from build123d import *

# Parameters (mm, degrees)
SKETCH042_R       = 4
PAD018_DEPTH      = 18.8
SKETCH045_R       = 3.3
PAD019_DEPTH      = 8
SKETCH050_R       = 4
PAD021_DEPTH      = 33.8
CYLINDER003_R     = 3.3
CYLINDER003_DEPTH = 8


with BuildPart() as part:
    # Sketch042 (on DatumPlane) → Pad018 (new body)
    with BuildSketch(Plane(origin=(0, 0, 18.8), x_dir=(0, 1, 0), z_dir=(0, 0, 1))):
        Circle(SKETCH042_R)
    extrude(amount=-PAD018_DEPTH)

    # Sketch045 (on Face2 of Pad018) → Pad019 (join)
    with BuildSketch(Plane(origin=(0, 0, 18.8), x_dir=(0, 1, 0), z_dir=(0, 0, 1))):
        Circle(SKETCH045_R)
    extrude(amount=PAD019_DEPTH)

    # Sketch050 (on Face3 of Pad019) → Pad021 (join)
    with BuildSketch(Plane.YX):
        Circle(SKETCH050_R)
    extrude(amount=PAD021_DEPTH)

    # Cylinder003 → Cylinder003 (join)
    with BuildSketch(Plane.YX.offset(33.8)):
        Circle(CYLINDER003_R)
    extrude(amount=CYLINDER003_DEPTH)


solid = part.part
Can you work these out from the model? Positions are in its coordinate system, mm. A direction names the side the tool comes from. Give positions to 0.01 mm unless a question says otherwise; leave off trailing zeros. Loops run counter-clockwise (first coordinate to the right, second up) from the corner with the lowest first, then second, coordinate; pieces in that order, holes last. Notation, with made-up numbers: (10, 0.25) - (29, 0.25) arc R27 ccw to (29, 31.25) - close; hole circle Ø11 at (7, -34). An arc over 180 degrees is marked (long way). Return JSON: item names as keys, results as strings.
1. I want a section at A-A on x = 0. Please give me the cut outline in (y, z), and give its area (3 significant figures).
Output values:
{"outline": "(-4, -33.8) - (-3.3, -33.8) - (-3.3, -41.8) - (3.3, -41.8) - (3.3, -33.8) - (4, -33.8) - (4, 18.8) - (3.3, 18.8) - (3.3, 26.8) - (-3.3, 26.8) - (-3.3, 18.8) - (-4, 18.8) - close", "area": "526 mm²"}
2. I'm going to push flat-ended pins straight in: pin 1 Ø3 at (y, z) = (-2.5, 4.5) entering from -X; pin 2 Ø3 at (x, z) = (-2, -25) entering from -Y. Where does each tip first touch, or does it pass through?
Output values:
{"pin 1": "stops at x = -3.87", "pin 2": "stops at y = -3.97"}
3. I want a section at C-C on z = -13.5. Please give me the cut outline in (x, y).
Output values:
{"outline": "circle Ø8 at (0, 0)"}
4. If I drill on line 1 (Z direction, x = -2, y = -3.25); line 2 (X direction, y = 0.25, z = -14); line 3 (X direction, y = 2.25, z = -31), over which ranges is the centre line in solid material (lowest first)?
Output values:
{"line 1": "z = -33.8 to 18.8", "line 2": "x = -3.99 to 3.99", "line 3": "x = -3.31 to 3.31"}
5. For faces 1 (the face through (-2.23, -2.43, 22.74)), 2 (the face through (0, 0, -41.8)), 3 (the face through (3, -2, -33.8)), which set-ups out of +Z, -Z, +X, -X, +Y, -Y let a thin tool reach every point of the face, with its end or its side?
Output values:
{"face 1": "+Z", "face 2": "-Z, +X, -X, +Y, -Y", "face 3": "-Z"}
